from build123d import *

# Parameters (mm, degrees)
SKETCH_1_R               = 4
SKETCH_1_R_2             = 3
EXTRUDE_1_DEPTH          = 6
EXTRUDE_START            = -1.5
SKETCH_2_R               = 16.5
SKETCH_2_R_2             = 4
EXTRUDE_2_DEPTH          = 1.5
SKETCH_4_R               = 0.75
CUT_EXTRUDE_1_DEPTH      = 1.5
PATTERN_CIRCULAR_1_COUNT = 8


with BuildPart() as part:
    # 草图1 → 凸台-拉伸1 (new body)
    with BuildSketch(Plane.XY):
        Circle(SKETCH_1_R)
        Circle(SKETCH_1_R_2, mode=Mode.SUBTRACT)
    extrude(amount=EXTRUDE_1_DEPTH)

    # 草图2 → 凸台-拉伸2 (add)
    with BuildSketch(Plane.XY.offset(6).offset(EXTRUDE_START)):
        Circle(SKETCH_2_R)
        Circle(SKETCH_2_R_2, mode=Mode.SUBTRACT)
    extrude(amount=EXTRUDE_2_DEPTH)

    # 草图4 → 切除-拉伸1 (cut)
    with BuildSketch(Plane.XY.offset(6)):
        with Locations((0, 14)):
            Circle(SKETCH_4_R)
        with Locations((0, 11.5)):
            Circle(SKETCH_4_R)
    cut_extrude_1 = extrude(amount=-CUT_EXTRUDE_1_DEPTH, mode=Mode.SUBTRACT)

    # 阵列(圆周)1: 切除-拉伸1 ×8 about axis
    pattern_circular_1_axis = Axis((0, 0, 4.5), (0, 0, 1))
    for i in range(1, PATTERN_CIRCULAR_1_COUNT):
        add(cut_extrude_1.rotate(pattern_circular_1_axis, i * 360 / PATTERN_CIRCULAR_1_COUNT), mode=Mode.SUBTRACT)


solid = part.part
Could you check a few things on this model? Use its own coordinates, in mm. Coordinates: 2 decimals unless noted, no trailing zeros. Order: outer loops, then holes, each group sorted by start corner. A loop starts at its lowest first (then second) coordinate and runs counter-clockwise, first axis right, second up. Notation, with made-up numbers: (74.5, 47.5) - (121.5, 47.5) arc R24 cw to (121.5, 81.5) - close; hole circle Ø8 at (-39, 76). An arc over 180 degrees is marked (long way). Answer in a Markdown table with one row per item. Add a question column.
(1) If we mould it in two halves opening along X, with no side actions, what happens to faces 1 (the face through (9.674, 9.184, 5.26)), 2 (the face through (-0.867, -3.905, 2.218)), 3 (the face through (3, -3, 4.5))? For each: released by +X, released by -X, zero draft, split by the parting line, or undercut.
(2) If we section it at B-B, the plane y = -11.5: Please give me the cut outline in (x, z), then the cut area to 3 significant figures.
(3) I need wall thicknesses on L1, parallel to Y at x = 0, z = 5.2; L2, parallel to Y at x = -0.5, z = 5.4; L3, parallel to Z at x = -7, y = -13.5. Which ranges of each line are inside material? Lowest first, please.
(4) If we section it at C-C, the plane x = -14: Please give me the cut outline in (y, z), then the cut area to 3 significant figures.
(5) If we section it at D-D, the plane z = 1.1: Please give me the cut outline in (x, y), then the cut area to 3 significant figures.
(6) Will this pin go through, and if not, where does the flat tip stop? pin 1 (5 mm diameter, centred on x = -0.5, y = -12.5, fed in from -Z).
(7) If we section it at A-A, the plane x = 0: Please give me the cut outline in (y, z).
Results are:
| question | item | result |
|---|---|---|
| 1 | face 1 | undercut |
| 1 | face 2 | split by the parting line |
| 1 | face 3 | zero draft |
| 2 | outline | (-11.83, 4.5) - (-0.75, 4.5) - (-0.75, 6) - (-11.83, 6) - close; (0.75, 4.5) - (11.83, 4.5) - (11.83, 6) - (0.75, 6) - close |
| 2 | area | 33.2 mm2 |
| 3 | L1 | y = -16.5 to -14.75, -13.25 to -12.25, -10.75 to -3, 3 to 10.75, 12.25 to 13.25, 14.75 to 16.5 |
| 3 | L2 | y = -16.49 to -14.56, -13.44 to -12.06, -10.94 to -2.96, 2.96 to 10.94, 12.06 to 13.44, 14.56 to 16.49 |
| 3 | L3 | z = 4.5 to 6 |
| 4 | outline | (-8.73, 4.5) - (-0.75, 4.5) - (-0.75, 6) - (-8.73, 6) - close; (0.75, 4.5) - (8.73, 4.5) - (8.73, 6) - (0.75, 6) - close |
| 4 | area | 23.9 mm2 |
| 5 | outline | circle Ø8 at (0, 0); hole circle Ø6 at (0, 0) |
| 5 | area | 22.0 mm2 |
| 6 | pin 1 | stops at z = 4.5 |
| 7 | outline | (-16.5, 4.5) - (-14.75, 4.5) - (-14.75, 6) - (-16.5, 6) - close; (-13.25, 4.5) - (-12.25, 4.5) - (-12.25, 6) - (-13.25, 6) - close; (-10.75, 4.5) - (-4, 4.5) - (-4, 0) - (-3, 0) - (-3, 6) - (-10.75, 6) - close; (3, 0) - (4, 0) - (4, 4.5) - (10.75, 4.5) - (10.75, 6) - (3, 6) - close; (12.25, 4.5) - (13.25, 4.5) - (13.25, 6) - (12.25, 6) - close; (14.75, 4.5) - (16.5, 4.5) - (16.5, 6) - (14.75, 6) - close |
